Autodesk Inventor part; units mm, degrees
ref_plane "YZ Plane" through (0, 0, 0) normal (1, 0, 0) x (0, 1, 0)
ref_plane "XZ Plane" through (0, 0, 0) normal (0, 1, 0) x (-1, 0, 0)
ref_plane "XY Plane" through (0, 0, 0) normal (0, 0, 1) x (1, 0, 0)
sketch "Sketch1" plane through (0, 0, 0) normal (0, 0, 1) x (1, 0, 0)
  line L0 (320, 0) -> (320, 670)
  line L1 (320, 670) -> (-480, 670)
  line L2 (-480, 670) -> (-480, 0)
  circle A0 centre (0, 350) radius 40
  line L3 (320, 0) -> (-480, 0)
  point P0 (0, 0)
  dimension "d14" = 80
  dimension "d15" = 320
  dimension "d17" = 320
  dimension "d26" = 800
  dimension "d27" = 670
extrude "Plate1" add sketch "Sketch1" along normal blind 3
sketch "Sketch2" plane through (0, 0, 0) normal (0, 0, -1) x (-1, 0, 0)
  line L0 (-300, 650) -> (-100, 650) construction
  line L1 (-100, 650) -> (-100, 630) construction
  line L2 (-100, 630) -> (-300, 630) construction
  line L3 (-300, 630) -> (-300, 650) construction
  line L4 (-320, 670) -> (480, 670)
  line L5 (-320, 0) -> (-320, 670)
  point P0 (0, 0)
  point P1 (-48, 100)
  point P2 (480, 670)
  point P3 (-251, -525)
  point P4 (-50, 98)
  point P5 (-320, 0)
  dimension "d6" = 200
  dimension "d9" = 20
  dimension "d10" = 20
  dimension "d11" = 20
mark "Mark1"
sketch "Sketch3" plane through (0, 0, 3) normal (0, 0, 1) x (1, 0, 0)
  circle A0 centre (0, 405) radius 5
  circle A1 centre (0, 350) radius 40
  point P0 (0, 0)
  dimension "d19" = 10
  dimension "d20" = 55
extrude "Cut1" cut sketch "Sketch3" against normal through all contours A0
pattern_circular "Circular Pattern1" count 6 over 360 about axis through (0, 350, 0) along (0, 0, 1) of "Cut1"
equation "\"d2\" = Thickness"
equation "\"BendReliefWidth\" = Thickness"
equation "\"BendReliefDepth\" = 0.5 * Thickness"
equation "\"CornerReliefSize\" = 4 * Thickness"
equation "\"MinimumRemnant\" = 2 * Thickness"
equation "\"TransitionRadius\" = BendRadius"
equation "\"JacobiRadiusSize\" = BendRadius"
equation "\"GapSize\" = Thickness"
properties part number "TRM 015 left board main" material "AISI 304"
Could you check a few things on this model? Use its own coordinates, in mm. Give positions to 0.01 mm unless a question says otherwise; leave off trailing zeros. Loops run counter-clockwise (first coordinate to the right, second up) from the corner with the lowest first, then second, coordinate; pieces in that order, holes last. Notation, with made-up numbers: (41.25, 17) - (49.25, 17) arc R29 ccw to (49.25, 51) - close; hole circle Ø10 at (-36, 33.25). An arc over 180 degrees is marked (long way). Answer in a Markdown table with one row per item. Add a question column.
Q1. Please list where these lines run through material, in increasing order: L1, parallel to Y at x = 0, z = 0.9; L2, parallel to X at y = 295, z = 0.7; L3, parallel to X at y = 292.5, z = 0.2. Write a range as from..to.
Q2. If we section it at A-A (y = 350): List the corners of the cut face in (x, z) for me.
Q3. We'd pull the mould along Y, two halves only. Please class faces 1 (the face through (-86, 340, 3)), 2 (the face through (-5.21, 310.34, 1.48)): +Y half, -Y half, draft (parallel to the pull), parting line (faces both ways), or undercut.
The answers:
| question | item | result |
|---|---|---|
| 1 | L1 | y = 0..290, 300..310, 390..400, 410..670 |
| 1 | L2 | x = -480..-5, 5..320 |
| 1 | L3 | x = -480..-4.33, 4.33..320 |
| 2 | outline | (-480, 0) - (-40, 0) - (-40, 3) - (-480, 3) - close; (40, 0) - (320, 0) - (320, 3) - (40, 3) - close |
| 3 | face 1 | draft |
| 3 | face 2 | undercut |
